Can you work these out from the model? Positions are in its coordinate system, mm. A direction names the side the tool comes from. Coordinates: 2 decimals unless noted, no trailing zeros. Loops run counter-clockwise (first coordinate to the right, second up) from the corner with the lowest first, then second, coordinate; pieces in that order, holes last. Notation, with made-up numbers: (1, 49.5) -> (46, 49.5) arc R27 ccw to (46, 80.5) -> close; hole circle Ø9 at (-35, 68). An arc over 180 degrees is marked (long way). Use one line per item in the form item = value. Start each with the question number.
(1) I need wall thicknesses on line 1 (X direction, y = 0.6, z = -62); line 2 (X direction, y = 0.3, z = 34); line 3 (X direction, y = 0.1, z = -7.5). Which ranges of each line are inside material? Lowest first, please. Write a range as [from, to].
(2) Imagine slicing it at D-D (x = 50). List the corners of the cut face in (y, z) for me.
(3) On a 3-axis mill with a long thin cutter (end or side, diameter ignored), from which of +Z, -Z, +X, -X, +Y, -Y can I reach the whole of each face in a straight line? I mean faces 1 (the flat face through (42.763, 0.493, 15.21)), 2 (the cylindrical face through (3.06, 0.49, 36.29)). Say none if no direction works.
(4) Imagine slicing it at C-C (y = 0.7). State how many separate pieces and enclosed holes the cut face has, plus the area to 3 significant figures.
(5) Imagine slicing it at B-B (x = 12). List the corners of the cut face in (y, z) for me, plus the area to 3 significant figures.
(6) Imagine slicing it at A-A (z = -21.5). List the corners of the cut face in (x, y) for me.
(7) I'm going to push a flat-ended pin straight in: pin 1 (1.8 mm diameter, centred on x = 0, z = 0, fed in from +Y). Where does the tip first touch, or does it pass through?
(8) Thinking about a two-plate mould opening in X: for faces 3 (the flat face through (46, 1, -31)), 4 (the cylindrical face through (46.983, 0.493, 36.251)), 5 (the cylindrical face through (48.536, 0.493, -0.325)), 6 (the flat face through (-0.433, 0.493, 17.674)), which applies, released by +X, released by -X, zero draft, split by the parting line, or undercut?
```python
from build123d import *

# Parameters (mm, degrees)
SKETCH_1_R      = 1.5
EXTRUDE_1_DEPTH = 1


with BuildPart() as part:
    # 草图1 → 凸台-拉伸1 (new body)
    with BuildSketch(Plane(origin=(0, 0, 0), x_dir=(1, 0, 0), z_dir=(0, 1, 0))):
        with BuildLine():
            Line((5, 99), (45, 99))
            ThreePointArc((45, 99), (46.960937797, 98.270401497), (47.968077406, 96.436481971))
            Line((47.968077406, 96.436481971), (52.968077406, 62.436481971))
            ThreePointArc((52.968077406, 62.436481971), (52.992008708, 62.218823881), (53, 62))
            Line((53, 62), (53, 0))
            ThreePointArc((53, 0), (52.992008708, -0.218823881), (52.968077406, -0.436481971))
            Line((52.968077406, -0.436481971), (47.968077406, -34.436481971))
            ThreePointArc((47.968077406, -34.436481971), (46.960937797, -36.270401497), (45, -37))
            Line((45, -37), (5, -37))
            ThreePointArc((5, -37), (3.039062203, -36.270401497), (2.031922594, -34.436481971))
            Line((2.031922594, -34.436481971), (-2.968077406, -0.436481971))
            ThreePointArc((-2.968077406, -0.436481971), (-2.992008708, -0.218823881), (-3, 0))
            Line((-3, 0), (-3, 62))
            ThreePointArc((-3, 62), (-2.992008708, 62.218823881), (-2.968077406, 62.436481971))
            Line((-2.968077406, 62.436481971), (2.031922594, 96.436481971))
            ThreePointArc((2.031922594, 96.436481971), (3.039062203, 98.270401497), (5, 99))
        make_face()
        with Locations(Location((0, 62, 0), (0, 0, 270))):
            Circle(SKETCH_1_R, mode=Mode.SUBTRACT)
        with Locations(Location((50, 62, 0), (0, 0, 270))):
            Circle(SKETCH_1_R, mode=Mode.SUBTRACT)
        with Locations(Location((0, 0, 0), (0, 0, 270))):
            Circle(SKETCH_1_R, mode=Mode.SUBTRACT)
        with Locations(Location((50, 0, 0), (0, 0, 270))):
            Circle(SKETCH_1_R, mode=Mode.SUBTRACT)
        with Locations(Location((5, 96, 0), (0, 0, 270))):
            Circle(SKETCH_1_R, mode=Mode.SUBTRACT)
        with Locations(Location((45, 96, 0), (0, 0, 270))):
            Circle(SKETCH_1_R, mode=Mode.SUBTRACT)
        with Locations(Location((5, -34, 0), (0, 0, 270))):
            Circle(SKETCH_1_R, mode=Mode.SUBTRACT)
        with Locations(Location((45, -34, 0), (0, 0, 270))):
            Circle(SKETCH_1_R, mode=Mode.SUBTRACT)
        Polygon((9.411764706, 92), (5, 62), (5, 0), (9.411764706, -30), (40.588235294, -30), (45, 0), (45, 62), (40.588235294, 92), align=None, mode=Mode.SUBTRACT)
    extrude(amount=EXTRUDE_1_DEPTH)


solid = part.part
```
Worked out:
q1.line_1 = [-3, -1.5], [1.5, 5], [45, 48.5], [51.5, 53]
q1.line_2 = [1.97, 3.5], [6.5, 43.5], [46.5, 48.03]
q1.line_3 = [-3, 5], [45, 53]
q2.outline = (0, -82.62) -> (1, -82.62) -> (1, -63.5) -> (0, -63.5) -> close; (0, -60.5) -> (1, -60.5) -> (1, -1.5) -> (0, -1.5) -> close; (0, 1.5) -> (1, 1.5) -> (1, 20.62) -> (0, 20.62) -> close
q3.face_1 = +Y, -Y
q3.face_2 = +Z, -X, +Y, -Y
q4.separate_pieces = 1
q4.enclosed_holes = 9
q4.area = 2,540 mm2
q5.outline = (0, -99) -> (1, -99) -> (1, -92) -> (0, -92) -> close; (0, 30) -> (1, 30) -> (1, 37) -> (0, 37) -> close
q5.area = 14.0 mm2
q6.outline = (-3, 0) -> (5, 0) -> (5, 1) -> (-3, 1) -> close; (45, 0) -> (53, 0) -> (53, 1) -> (45, 1) -> close
q7.pin_1 = through
q8.face_3 = zero draft
q8.face_4 = released by +X
q8.face_5 = undercut
q8.face_6 = released by -X
